Work out the finished part from the listing and answer in its coordinate system (mm). A direction names the side the tool comes from. Coordinates: 2 decimals unless noted, no trailing zeros. Write each loop counter-clockwise with the first axis right and the second up, starting at its lowest first coordinate (ties: lowest second). Pieces come first, ordered by that corner, then holes. Notation, with made-up numbers: (-23, -30) - (-16, -30) arc R18 ccw to (-16, 2) - close; hole circle Ø6 at (66, 7.5). An arc over 180 degrees is marked (long way). Use one line per item in the form item = value. Start each with the question number.
Item 1: A cutting plane is placed at A-A (y = 6). Write down the section's boundary in (x, z), then the cut area to 3 significant figures.
Item 2: For faces 1 (the flat face through (22.5, 0, 6)), 2 (the flat face through (45, -8, -20)), 3 (the flat face through (-10.106, 17.836, 15.986)), 4 (the flat face through (-20.5, 0, 16)), 5 (the flat face through (-10.394, -17.671, 15.986)), determine the directions among +Z, -Z, +X, -X, +Y, -Y from which every point of the face is accessible in a straight line to the end or side of a thin tool.
Item 3: A cutting plane is placed at B-B (z = 4). Write down the section's boundary in (x, y).
Item 4: A cutting plane is placed at D-D (y = -4). Write down the section's boundary in (x, z), then the cut area to 3 significant figures.
Item 5: Consider probe 1 along X at (y, z) = (7, 2.5); probe 2 along X at (y, z) = (-4, -18.5); probe 3 along Z at (x, y) = (-1, -14). Determine where each line is inside the solid, lowest interval first.
Item 6: Given pin 1 (8 mm diameter, centred on y = -2.5, z = -43.5, fed in from -X); pin 2 (13.5 mm diameter, centred on x = 9, y = 6, fed in from -Z); pin 3 (3 mm diameter, centred on x = 13.5, y = 19, fed in from -Z), each flat-ended and moving along its own axis, determine where each tip first touches the part or whether it passes through.
Item 7: A cutting plane is placed at C-C (x = 31.5). Write down the section's boundary in (y, z).
from build123d import *

# Parameters (mm, degrees)
BOSS_EXTRUDE1_DEPTH = 15
BOSS_EXTRUDE2_DEPTH = 2
FILLET1_R           = 3
SKETCH3_W           = 56
SKETCH3_H           = 8
BOSS_EXTRUDE3_DEPTH = 6
SKETCH4_W           = 12
SKETCH4_H           = 8
BOSS_EXTRUDE4_DEPTH = 45
SKETCH5_R           = 3.5
BOSS_EXTRUDE5_DEPTH = 11
FILLET2_R           = 4


with BuildPart() as part:
    # Sketch1 → Boss-Extrude1 (new body)
    with BuildSketch(Plane.XY):
        Polygon((0, 25.980762114), (-22.5, 12.990381057), (-22.5, -12.990381057), (0, -25.980762114), (22.5, -12.990381057), (22.5, 12.990381057), align=None)
    extrude(amount=BOSS_EXTRUDE1_DEPTH)

    # Sketch2 → Boss-Extrude2 (add)
    with BuildSketch(Plane.XY.offset(15)):
        Polygon((20.5, 11.835680518), (0, 23.671361037), (-20.5, 11.835680518), (-20.5, -11.835680518), (0, -23.671361037), (20.5, -11.835680518), align=None)
    extrude(amount=BOSS_EXTRUDE2_DEPTH)

    # Fillet1
    # the kernel refuses this fillet: 3 mm, written as the material it takes off along each edge
    with BuildSketch(Plane(origin=(-22.5, 20.061448869, 15), x_dir=(0, 0, -1), z_dir=(0, -1, 0)), Plane(origin=(28.623724357, 9.454847151, 15), x_dir=(0, 0, -1), z_dir=(-0.8660254037844388, 0.4999999999999997, 0)), Plane(origin=(6.123724357, 29.516296019, 15), x_dir=(0, 0, -1), z_dir=(-0.8660254037844386, -0.5000000000000003, 0))) as fillet1_piece_1:
        with BuildLine():
            CenterArc((2.828427125, 3), FILLET1_R, 199.471220634, 70.528779366)
            Line((0, 2), (-0.056568542, 1.98))
            ThreePointArc((-0.056568542, 1.98), (-0.06, 1), (-0.06, 0))
            Line((-0.06, 0), (0, -0.06))
            Line((0, -0.06), (2.828427125, -0.06))
            Line((2.828427125, -0.06), (2.828427125, 0))
        make_face()
    extrude(amount=40.122897737, mode=Mode.SUBTRACT)
    with BuildSketch(Plane(origin=(-28.623724357, -9.454847151, 15), x_dir=(0.5000000000000002, 0.8660254037844386, 0), z_dir=(0.8660254037844386, -0.5000000000000002, 0)), Plane(origin=(-6.123724357, -29.516296019, 15), x_dir=(-0.5000000000000003, 0.8660254037844386, 0), z_dir=(0.8660254037844385, 0.5000000000000003, 0)), Plane(origin=(22.5, -20.061448869, 15), x_dir=(-1, 0, 0), z_dir=(0, 1, 0))) as fillet1_piece_2:
        with BuildLine():
            CenterArc((3, -2.828427125), FILLET1_R, 109.471220634, 70.528779366)
            Line((0, -2.828427125), (-0.06, -2.828427125))
            Line((-0.06, -2.828427125), (-0.06, 0))
            Line((-0.06, 0), (0, 0.06))
            ThreePointArc((0, 0.06), (1, 0.06), (1.98, 0.056568542))
            Line((1.98, 0.056568542), (2, 0))
        make_face()
    extrude(amount=40.122897737, mode=Mode.SUBTRACT)

    # Sketch3 → Boss-Extrude3 (add)
    with BuildSketch(Plane(origin=(0, 0, 0), x_dir=(-1, 0, 0), z_dir=(0, 0, -1))):
        with Locations((-28, -4)):
            Rectangle(SKETCH3_W, SKETCH3_H)
    extrude(amount=BOSS_EXTRUDE3_DEPTH)

    # Sketch4 → Boss-Extrude4 (add)
    with BuildSketch(Plane(origin=(0, 0, -6), x_dir=(-1, 0, 0), z_dir=(0, 0, -1))):
        with Locations((-50, -4)):
            Rectangle(SKETCH4_W, SKETCH4_H)
    extrude(amount=BOSS_EXTRUDE4_DEPTH)

    # Sketch5 → Boss-Extrude5 (add)
    with BuildSketch(Plane(origin=(56, 0, 0), x_dir=(0, 0, -1), z_dir=(1, 0, 0))):
        with Locations(Location((45, -4, 0), (0, 0, 180))):
            Circle(SKETCH5_R)
    extrude(amount=BOSS_EXTRUDE5_DEPTH)

    # Fillet2
    fillet2_edges = [part.edges().sort_by_distance(p)[0] for p in [
        (0, -4, -6),
    ]]
    fillet(fillet2_edges, radius=FILLET2_R)


solid = part.part
Answer:
q1.outline = (-22.5, 0) - (22.5, 0) - (22.5, 12.17) arc R3 ccw to (20.5, 15) - (20.5, 17) - (-20.5, 17) - (-20.5, 15) arc R3 ccw to (-22.5, 12.17) - close
q1.area = 754 mm²
q2.face_1 = +Z, +X, +Y, -Y
q2.face_2 = -Z, +X, -X, -Y
q2.face_3 = +Z, -X, +Y
q2.face_4 = +Z, -X, +Y, -Y
q2.face_5 = +Z, -X, -Y
q3.outline = (-22.5, -12.99) - (0, -25.98) - (22.5, -12.99) - (22.5, 12.99) - (0, 25.98) - (-22.5, 12.99) - close
q4.outline = (-22.5, 0) - (0, 0) - (0, -2) arc R4 ccw to (4, -6) - (44, -6) - (44, -51) - (56, -51) - (56, -48.5) - (67, -48.5) - (67, -41.5) - (56, -41.5) - (56, 0) - (22.5, 0) - (22.5, 12.17) arc R3 ccw to (20.5, 15) - (20.5, 17) - (-20.5, 17) - (-20.5, 15) arc R3 ccw to (-22.5, 12.17) - close
q4.area = 1,700 mm²
q5.probe_1 = -22.5 to 22.5
q5.probe_2 = 44 to 56
q5.probe_3 = 0 to 17
q6.pin_1 = 44
q6.pin_2 = -6
q6.pin_3 = 0
q7.outline = (-8, -6) - (0, -6) - (0, 0) - (-8, 0) - close
